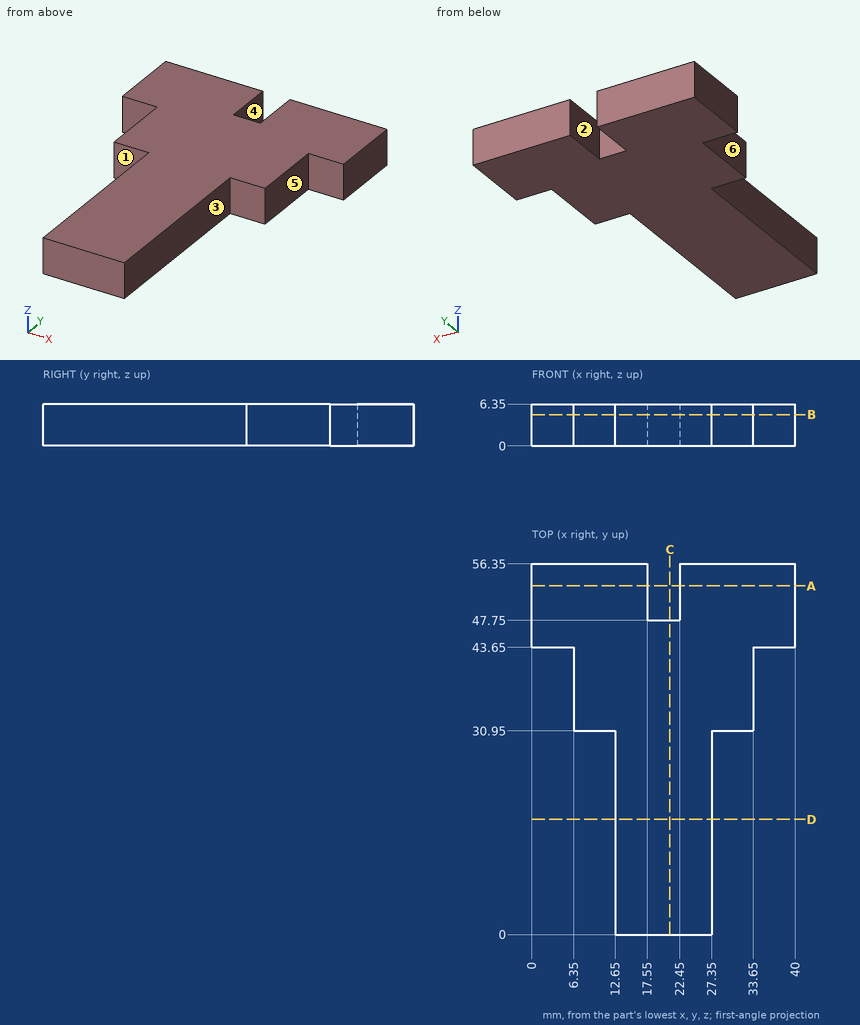
Verification items for this drawing (mm, ordinates from the low corner). A direction names the side the tool comes from. Coordinates: 2 decimals unless noted, no trailing zeros. Write each loop counter-clockwise with the first axis right and the second up, starting at its lowest first coordinate (ties: lowest second). Pieces come first, ordered by that corner, then holes. Notation, with made-up numbers: M 66.25,67 L 107.25,67 A23 cw 107.25,106 Z; hole C 45,10 d7. An arc over 180 degrees is marked long. Answer as a JSON object with one key per item and string values. Group by question number.
(1) Tool access check on the marked faces 4, 5 and 6. Record the directions out of +Z, -Z, +X, -X, +Y, -Y that give a thin tool (end or side, any length) a straight path to the whole face; none if there is none.
(2) Gauge pin test, flat ends, axial feed: pin 1 (3 mm diameter, centred on y = 35, z = 4.5, fed in from -X); pin 2 (3 mm diameter, centred on x = 35.5, z = 2.5, fed in from -Y); pin 3 (1 mm diameter, centred on y = 16, z = 2, fed in from +X). Record the tip position at first contact, or that the pin passes through.
(3) Cross-section at B-B, the plane z = 4.75. Record the cut outline in (x, y), and give its area (3 significant figures).
(4) Cross-section at C-C, the plane x = 21. Record the cut outline in (y, z).
(5) Release check for a two-part mould opening along X. For the marked faces 1, 2 and 3 record: +X half, -X half, draft (parallel to the pull), parting line (faces both ways), or undercut.
(6) Cross-section at D-D, the plane y = 17.5. Record the cut outline in (x, z), and give its area (3 significant figures).
(7) Material ranges on line 1 (X direction, y = 52.5, z = 0.75); line 2 (X direction, y = 35.5, z = 1.5); line 3 (Y direction, x = 18.5, z = 3.75), recorded low to high.
(8) Cross-section at A-A, the plane y = 53. Record the cut outline in (x, z).
Reply:
{
 "1": {"face 4": "+Z, -Z, +Y", "face 5": "+Z, -Z, +X, -Y", "face 6": "+Z, -Z, -X, -Y"},
 "2": {"pin 1": "x = 6.35", "pin 2": "y = 43.65", "pin 3": "x = 27.35"},
 "3": {"outline": "M 0,43.65 L 6.35,43.65 L 6.35,30.95 L 12.65,30.95 L 12.65,0 L 27.35,0 L 27.35,30.95 L 33.65,30.95 L 33.65,43.65 L 40,43.65 L 40,56.35 L 22.45,56.35 L 22.45,47.75 L 17.55,47.75 L 17.55,56.35 L 0,56.35 Z", "area": "1,270 mm²"},
 "4": {"outline": "M 0,0 L 47.75,0 L 47.75,6.35 L 0,6.35 Z"},
 "5": {"face 1": "draft", "face 2": "undercut", "face 3": "+X half"},
 "6": {"outline": "M 12.65,0 L 27.35,0 L 27.35,6.35 L 12.65,6.35 Z", "area": "93.3 mm²"},
 "7": {"line 1": "0 to 17.55, 22.45 to 40", "line 2": "6.35 to 33.65", "line 3": "0 to 47.75"},
 "8": {"outline": "M 0,0 L 17.55,0 L 17.55,6.35 L 0,6.35 Z; M 22.45,0 L 40,0 L 40,6.35 L 22.45,6.35 Z"}
}
